CAD build for the part. Positions are in the model's coordinates, mm. Face numbers are marked on the shaded views. A direction names the side the tool comes from. Give positions to 0.01 mm unless a question says otherwise; leave off trailing zeros. Write each loop counter-clockwise with the first axis right and the second up, starting at its lowest first coordinate (ties: lowest second). Pieces come first, ordered by that corner, then holes. Notation, with made-up numbers: (19, 42) - (57, 42) arc R11 ccw to (57, 62) - close; hole circle Ø5 at (64.25, 76). An arc over 180 degrees is marked (long way). Put each result on its own line as item: value. Start each with the question number.
1. Cut at A-A on z = 0. Give the number of separate pieces and of enclosed holes in the cut face, and give its area (3 significant figures).
2. Tool access for the marked faces 4 and 5: list every direction of +Z, -Z, +X, -X, +Y, -Y with a clear straight run to the whole face (end or side of a thin tool).
3. Mould opens along Y. For the marked faces 1, 2 and 3 say: +Y half, -Y half, draft (parallel to the pull), parting line (faces both ways), or undercut.
4. Wall check: line 1 (X direction, y = 1.5, z = 0); line 2 (Y direction, x = -53.5, z = -4.5); line 3 (X direction, y = 31, z = 11). Give the ranges that are in metal, low to high.
5. Cut at B-B on x = -32. List the corners of the cut face in (y, z), and give its area (3 significant figures).
6. Drop flat-ended pins along their axis: pin 1 (8 mm diameter, centred on x = 11.5, y = 32, fed in from +Z); pin 2 (1 mm diameter, centred on y = 23, z = -33.5, fed in from +X); pin 3 (6 mm diameter, centred on x = -23, y = 12.5, fed in from +Z). Give the stop position or say it passes through.
7. Cut at D-D on y = 15.5. List the corners of the cut face in (x, z) (1 decimal), and give its area (3 significant figures).
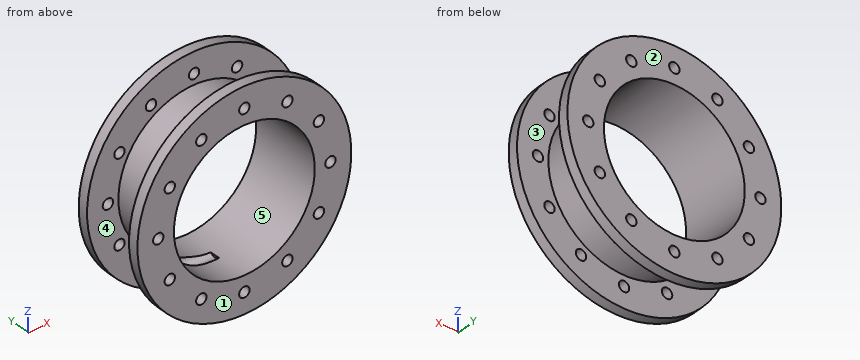
from build123d import *

# Parameters (mm, degrees)
SKETCH1_R            = 65.08749999999999
SKETCH1_R_2          = 3.1749999999997374
SKETCH1_R_3          = 3.174999999999826
SKETCH1_R_4          = 3.1749999999999874
SKETCH1_R_5          = 3.1749999999998075
SKETCH1_R_6          = 3.1749999999998435
SKETCH1_R_7          = 3.174999999999926
SKETCH1_R_8          = 3.1750000000000713
SKETCH1_R_9          = 3.1750000000002263
SKETCH1_R_10         = 3.1749999999999767
SKETCH1_R_11         = 3.175000000000085
SKETCH1_R_12         = 3.175000000000142
BOSS_EXTRUDE1_DEPTH  = 6.35
BOSS_EXTRUDE7_DEPTH  = 6.35
MOVE_FACE6_BY        = 6.35
MOVE_FACE6_2_BY      = 6.35
MOVE_FACE6_3_BY      = 6.35
BOSS_EXTRUDE8_START  = 44.449999999999996
BOSS_EXTRUDE8_DEPTH  = 44.449999999999996
BOSS_EXTRUDE10_START = 6.35
SKETCH1_13_R         = 65.08749999999999
SKETCH1_13_R_2       = 3.1749999999997374
SKETCH1_13_R_3       = 3.174999999999826
SKETCH1_13_R_4       = 3.1749999999999874
SKETCH1_13_R_5       = 3.1749999999998075
SKETCH1_13_R_6       = 3.1749999999998435
SKETCH1_13_R_7       = 3.174999999999926
SKETCH1_13_R_8       = 3.1750000000000713
SKETCH1_13_R_9       = 3.1750000000002263
SKETCH1_13_R_10      = 3.1749999999999767
SKETCH1_13_R_11      = 3.175000000000085
SKETCH1_13_R_12      = 3.175000000000142
BOSS_EXTRUDE10_DEPTH = 6.35
SKETCH2_R            = 4.49012806053458
CUT_EXTRUDE1_DEPTH   = 38.1


with BuildPart() as part:
    # Sketch1 → Boss-Extrude1 (new body)
    # profile 1 of 2: a face of its own
    with BuildSketch(Plane(origin=(0, 0, 0), x_dir=(1, 0, 0), z_dir=(0, 1, 0))):
        with Locations(Location((0, 0, 0), (0, 0, 270))):
            Circle(SKETCH1_R)
        with Locations(Location((-26.193749999999444, -45.36890584075757, 0), (0, 0, 270))):
            Circle(SKETCH1_R_2, mode=Mode.SUBTRACT)
        with Locations(Location((-45.36890584075695, -26.193750000000517, 0), (0, 0, 270))):
            Circle(SKETCH1_R_3, mode=Mode.SUBTRACT)
        with Locations(Location((-52.38749999999999, -5.8287e-13, 0), (0, 0, 270))):
            Circle(SKETCH1_R_4, mode=Mode.SUBTRACT)
        with Locations(Location((5.8437e-13, -52.38749999999999, 0), (0, 0, 270))):
            Circle(SKETCH1_R_5, mode=Mode.SUBTRACT)
        with Locations(Location((26.193750000000502, -45.368905840756966, 0), (0, 0, 270))):
            Circle(SKETCH1_R_6, mode=Mode.SUBTRACT)
        with Locations(Location((45.36890584075758, -26.193749999999447, 0), (0, 0, 270))):
            Circle(SKETCH1_R_7, mode=Mode.SUBTRACT)
        with Locations(Location((-45.36890584075756, 26.193749999999472, 0), (0, 0, 270))):
            Circle(SKETCH1_R_8, mode=Mode.SUBTRACT)
        with Locations(Location((-6.0368e-13, 52.38750000000001, 0), (0, 0, 270))):
            Circle(SKETCH1_R_9, mode=Mode.SUBTRACT)
        with BuildLine():
            Line((-24.244761862165653, 42.86249999999999), (-16.800520825261128, 42.8625))
            ThreePointArc((-16.80052082526106, 42.86249999999964), (25.94221876360081, 38.03225856916045), (46.0375, 0))
            ThreePointArc((46.0375, -1.128e-14), (-20.353392839950203, -41.29395604870844), (-28.040840750590878, 36.51250000000003))
            Line((-28.040840750590878, 36.51249999999999), (-38.10000000000001, 36.51249999999999))
            Line((-38.10000000000001, 36.51249999999999), (-38.10000000000001, 42.86249999999999))
            Line((-38.10000000000001, 42.86249999999999), (-28.142738137835213, 42.86249999999999))
            ThreePointArc((-28.142738137835213, 42.86249999999998), (-27.588846351937473, 48.2209807291169), (-23.01875000000034, 45.36890584075697))
            ThreePointArc((-23.01875000000034, 45.36890584075697), (-23.341675111640548, 43.973809488820095), (-24.24476186216568, 42.86250000000009))
        make_face(mode=Mode.SUBTRACT)
        with Locations(Location((52.38749999999997, 5.8711e-13, 0), (0, 0, 270))):
            Circle(SKETCH1_R_10, mode=Mode.SUBTRACT)
        with Locations(Location((45.36890584075695, 26.19375000000053, 0), (0, 0, 270))):
            Circle(SKETCH1_R_11, mode=Mode.SUBTRACT)
        with Locations(Location((26.19374999999944, 45.36890584075759, 0), (0, 0, 270))):
            Circle(SKETCH1_R_12, mode=Mode.SUBTRACT)
    # profile 2 of 2: a face of its own
    with BuildSketch(Plane(origin=(0, 0, 0), x_dir=(1, 0, 0), z_dir=(0, 1, 0))):
        with BuildLine():
            ThreePointArc((-28.040840750590878, 36.51250000000003), (-22.644371309313744, 40.08346110624591), (-16.80052082526106, 42.86249999999964))
            Line((-16.800520825261128, 42.8625), (-24.244761862165653, 42.86249999999999))
            ThreePointArc((-24.24476186216568, 42.86250000000009), (-26.19375000000043, 42.1939058407568), (-28.142738137835213, 42.86249999999998))
            Line((-28.142738137835213, 42.86249999999999), (-38.10000000000001, 42.86249999999999))
            Line((-38.10000000000001, 42.86249999999999), (-38.10000000000001, 36.51249999999999))
            Line((-38.10000000000001, 36.51249999999999), (-28.040840750590878, 36.51249999999999))
        make_face()
    extrude(amount=BOSS_EXTRUDE1_DEPTH)


with BuildPart() as part_1:
    # Move Face4: read off the stored shape, not the designer's step
    # Move Face4: moved
    add(part.part.moved(Location((0, 44.45, 0))))

    # Move Face6: a face moved outward by 6.35
    extrude(part_1.faces().sort_by_distance((-32.54375, 44.45, 52.07))[0], amount=MOVE_FACE6_BY, dir=(0, -1, 0))

    # Move Face6 2: a curved face moved outward by 6.35
    add(Solid.thicken(part_1.faces().sort_by_distance((0, 47.625, -65.0875))[0], -MOVE_FACE6_2_BY))

    # Move Face6 3: a face moved inward by 6.35
    extrude(part_1.faces().sort_by_distance((-32.54375, 50.8, 52.07))[0], amount=MOVE_FACE6_3_BY, dir=(0, -1, 0), mode=Mode.SUBTRACT)

    # Sketch1<11> → Boss-Extrude8 (add)
    with BuildSketch(Plane(origin=(0, 0, 0), x_dir=(1, 0, 0), z_dir=(0, 1, 0)).offset(BOSS_EXTRUDE8_START)):
        with BuildLine():
            ThreePointArc((-22.45064030267289, 36.512499999999996), (-11.66569490000489, 41.244459855233885), (2.62e-15, 42.8625))
            Line((0, 42.8625), (-16.800520825261128, 42.8625))
            ThreePointArc((-16.80052082526106, 42.86249999999964), (-22.644371309313744, 40.08346110624591), (-28.040840750590878, 36.51250000000003))
            Line((-28.040840750590878, 36.51249999999999), (-22.4506403026729, 36.51249999999999))
        make_face()
        with BuildLine():
            Line((-16.800520825261128, 42.8625), (0, 42.8625))
            ThreePointArc((2.62e-15, 42.8625), (30.308364408608394, 30.308364408608387), (42.8625, 0))
            ThreePointArc((42.8625, -1.05e-14), (-20.91534527896545, -37.41312922105898), (-22.45064030267289, 36.512499999999996))
            Line((-22.4506403026729, 36.51249999999999), (-28.040840750590878, 36.51249999999999))
            ThreePointArc((-28.040840750590878, 36.51250000000003), (-20.353392839950203, -41.29395604870844), (46.0375, -1.128e-14))
            ThreePointArc((46.0375, 0), (25.94221876360081, 38.03225856916045), (-16.80052082526106, 42.86249999999964))
        make_face()
    extrude(amount=-BOSS_EXTRUDE8_DEPTH)

    # Sketch1<13> → Boss-Extrude10 (add)
    # profile 1 of 2: a face of its own
    with BuildSketch(Plane(origin=(0, 0, 0), x_dir=(1, 0, 0), z_dir=(0, 1, 0)).offset(BOSS_EXTRUDE10_START)):
        with Locations(Location((0, 0, 0), (0, 0, 270))):
            Circle(SKETCH1_13_R)
        with Locations(Location((-26.193749999999444, -45.36890584075757, 0), (0, 0, 270))):
            Circle(SKETCH1_13_R_2, mode=Mode.SUBTRACT)
        with Locations(Location((-45.36890584075695, -26.193750000000517, 0), (0, 0, 270))):
            Circle(SKETCH1_13_R_3, mode=Mode.SUBTRACT)
        with Locations(Location((-52.38749999999999, -5.8287e-13, 0), (0, 0, 270))):
            Circle(SKETCH1_13_R_4, mode=Mode.SUBTRACT)
        with Locations(Location((5.8437e-13, -52.38749999999999, 0), (0, 0, 270))):
            Circle(SKETCH1_13_R_5, mode=Mode.SUBTRACT)
        with Locations(Location((26.193750000000502, -45.368905840756966, 0), (0, 0, 270))):
            Circle(SKETCH1_13_R_6, mode=Mode.SUBTRACT)
        with Locations(Location((45.36890584075758, -26.193749999999447, 0), (0, 0, 270))):
            Circle(SKETCH1_13_R_7, mode=Mode.SUBTRACT)
        with Locations(Location((-45.36890584075756, 26.193749999999472, 0), (0, 0, 270))):
            Circle(SKETCH1_13_R_8, mode=Mode.SUBTRACT)
        with Locations(Location((-6.0368e-13, 52.38750000000001, 0), (0, 0, 270))):
            Circle(SKETCH1_13_R_9, mode=Mode.SUBTRACT)
        with BuildLine():
            Line((-24.244761862165653, 42.86249999999999), (-16.800520825261128, 42.8625))
            ThreePointArc((-16.80052082526106, 42.86249999999964), (25.94221876360081, 38.03225856916045), (46.0375, 0))
            ThreePointArc((46.0375, -1.128e-14), (-20.353392839950203, -41.29395604870844), (-28.040840750590878, 36.51250000000003))
            Line((-28.040840750590878, 36.51249999999999), (-38.10000000000001, 36.51249999999999))
            Line((-38.10000000000001, 36.51249999999999), (-38.10000000000001, 42.86249999999999))
            Line((-38.10000000000001, 42.86249999999999), (-28.142738137835213, 42.86249999999999))
            ThreePointArc((-28.142738137835213, 42.86249999999998), (-27.588846351937473, 48.2209807291169), (-23.01875000000034, 45.36890584075697))
            ThreePointArc((-23.01875000000034, 45.36890584075697), (-23.341675111640548, 43.973809488820095), (-24.24476186216568, 42.86250000000009))
        make_face(mode=Mode.SUBTRACT)
        with Locations(Location((52.38749999999997, 5.8711e-13, 0), (0, 0, 270))):
            Circle(SKETCH1_13_R_10, mode=Mode.SUBTRACT)
        with Locations(Location((45.36890584075695, 26.19375000000053, 0), (0, 0, 270))):
            Circle(SKETCH1_13_R_11, mode=Mode.SUBTRACT)
        with Locations(Location((26.19374999999944, 45.36890584075759, 0), (0, 0, 270))):
            Circle(SKETCH1_13_R_12, mode=Mode.SUBTRACT)
    # profile 2 of 2: a face of its own
    with BuildSketch(Plane(origin=(0, 0, 0), x_dir=(1, 0, 0), z_dir=(0, 1, 0)).offset(BOSS_EXTRUDE10_START)):
        with BuildLine():
            ThreePointArc((-28.040840750590878, 36.51250000000003), (-22.644371309313744, 40.08346110624591), (-16.80052082526106, 42.86249999999964))
            Line((-16.800520825261128, 42.8625), (-24.244761862165653, 42.86249999999999))
            ThreePointArc((-24.24476186216568, 42.86250000000009), (-26.19375000000043, 42.1939058407568), (-28.142738137835213, 42.86249999999998))
            Line((-28.142738137835213, 42.86249999999999), (-38.10000000000001, 42.86249999999999))
            Line((-38.10000000000001, 42.86249999999999), (-38.10000000000001, 36.51249999999999))
            Line((-38.10000000000001, 36.51249999999999), (-28.040840750590878, 36.51249999999999))
        make_face()
    extrude(amount=-BOSS_EXTRUDE10_DEPTH)


with BuildPart() as body_2:
    # Sketch1<9> → Boss-Extrude7 (new body)
    with BuildSketch(Plane(origin=(0, 0, 0), x_dir=(1, 0, 0), z_dir=(0, 1, 0))):
        Polygon((0, 36.51249999999999), (0, 42.8625), (-38.10000000000001, 42.86249999999999), (-38.10000000000001, 36.51249999999999), align=None)
    extrude(amount=BOSS_EXTRUDE7_DEPTH)


with BuildPart() as body_2_1:
    # Move Face5: read off the stored shape, not the designer's step
    # Move Face5: moved
    add(body_2.part.moved(Location((0, 19.05, 0))))


with BuildPart() as cut_extrude1_tool:
    # Sketch2 → Cut-Extrude1 (new body)
    with BuildSketch(Plane.ZY.offset(38.10000000000001)):
        with Locations((-39.68749999999999, 22.225)):
            Circle(SKETCH2_R)
    extrude(amount=-CUT_EXTRUDE1_DEPTH)


with BuildPart() as part_2:
    add(part_1.part)

    # Cut-Extrude1: cut by cut_extrude1_tool
    add(cut_extrude1_tool.part, mode=Mode.SUBTRACT)


with BuildPart() as body_2_2:
    add(body_2_1.part)

    # Cut-Extrude1: cut by cut_extrude1_tool
    add(cut_extrude1_tool.part, mode=Mode.SUBTRACT)


solid = part_2.part
Report:
1. separate pieces: 6
1. enclosed holes: 0
1. area: 605 mm²
2. face 4: none
2. face 5: +Y, -Y
3. face 1: -Y half
3. face 2: +Y half
3. face 3: undercut
4. line 1: x = -65.09 to -55.56, -49.21 to -42.86, 42.86 to 49.21, 55.56 to 65.09
4. line 2: y = 0 to 6.35, 38.1 to 44.45
4. line 3: x = -44.7 to -41.43, 41.43 to 44.7
5. outline: (0, -56.68) - (6.35, -56.68) - (6.35, -33.1) - (38.1, -33.1) - (38.1, -56.68) - (44.45, -56.68) - (44.45, -28.52) - (0, -28.52) - close; (0, 28.52) - (44.45, 28.52) - (44.45, 56.68) - (38.1, 56.68) - (38.1, 33.1) - (6.35, 33.1) - (6.35, 56.68) - (0, 56.68) - close
5. area: 1,010 mm²
6. pin 1: stops at z = 45.42
6. pin 2: stops at x = 32.1
6. pin 3: stops at z = 41.47
7. outline: circle Ø92.1 at (0, 0); hole circle Ø85.7 at (0, 0)
7. area: 887 mm²
